```python
from build123d import *

# Parameters (mm, degrees)
F2_SIZE = 1
F3_R    = 1


with BuildPart() as f1:
    # F0 (on Front) → F1 (revolve)
    with BuildSketch(Plane.XZ):
        Polygon((7, 17.2), (2.1, 17.2), (2.1, 0), (4.1, 0), (4.1, 15.2), (7, 15.2), align=None)
    revolve(axis=Axis((0, 0, 8.6), (0, 0, 1)))

    # F2
    f2_edges = [f1.edges().sort_by_distance(p)[0] for p in [
        (-2.1, 0, 17.2),
        (-4.1, 0, 0),
    ]]
    chamfer(f2_edges, length=F2_SIZE)

    # F3
    f3_edges = [f1.edges().sort_by_distance(p)[0] for p in [
        (-7, 0, 17.2),
    ]]
    fillet(f3_edges, radius=F3_R)


solid = f1.part
```
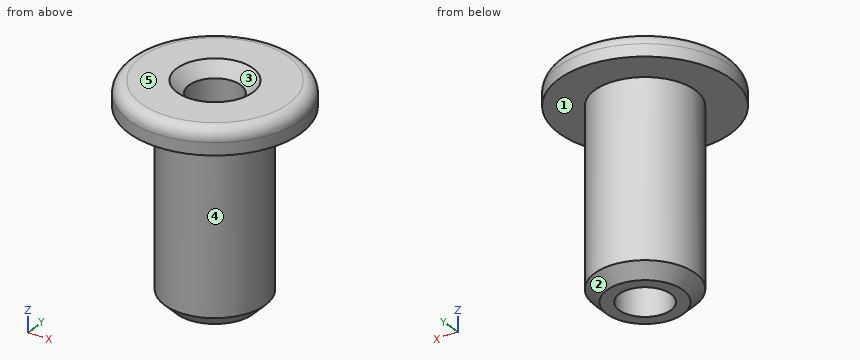
Input: part model. Units: mm. Frame: model coordinates. Face numbers are marked on the shaded views. A direction names the side the tool comes from. Give positions to 0.01 mm unless a question says otherwise; leave off trailing zeros. Order: outer loops, then holes, each group sorted by start corner. A loop starts at its lowest first (then second) coordinate and runs counter-clockwise, first axis right, second up. Notation, with made-up numbers: (-4.5, -1.5) - (54.5, -1.5) arc R12 cw to (54.5, 17.5) - close; hole circle Ø5 at (34.5, -15). An arc over 180 degrees is marked (long way). One line per item, written item: value.
1. Draft query along X for the marked faces 1, 2 and 3. Return one class per face: released by +X, released by -X, zero draft, split by the parting line, or undercut.
Determined:
face 1: zero draft
face 2: split by the parting line
face 3: undercut
2. Cut plane A-A, the plane y = 0. Output: boundary loops of the cut face in (x, z).
Determined:
outline: (-7, 15.2) - (-4.1, 15.2) - (-4.1, 1) - (-3.1, 0) - (-2.1, 0) - (-2.1, 16.2) - (-3.1, 17.2) - (-6, 17.2) arc R1 ccw to (-7, 16.2) - close; (2.1, 0) - (3.1, 0) - (4.1, 1) - (4.1, 15.2) - (7, 15.2) - (7, 16.2) arc R1 ccw to (6, 17.2) - (3.1, 17.2) - (2.1, 16.2) - close
3. Reachability of the marked faces 4 and 5 from +Z, -Z, +X, -X, +Y, -Y: full face, straight path, thin tool, end or side. Return the list, or none.
Determined:
face 4: -Z
face 5: +Z, +X, -X, +Y, -Y
4. Line query: probe 1 along Y at (x, z) = (0, 11.75); probe 2 along Z at (x, y) = (-2.5, -5.5); probe 3 along X at (y, z) = (1, 9.5). Output: solid intervals per line, ascending.
Determined:
probe 1: -4.1 to -2.1, 2.1 to 4.1
probe 2: 15.2 to 17.2
probe 3: -3.98 to -1.85, 1.85 to 3.98
5. Cut plane C-C, the plane z = 4.5. Output: boundary loops of the cut face in (x, y), and give its area (3 significant figures).
Determined:
outline: circle Ø8.2 at (0, 0); hole circle Ø4.2 at (0, 0)
area: 39.0 mm2
6. Pin query (flat end, axial travel): pin 1 Ø4 at (y, z) = (-2.5, 5) entering from -X; pin 2 Ø2 at (x, y) = (2, 0) entering from +Z; pin 3 Ø3 at (x, z) = (1.5, 2) entering from +Y. Return the tip coordinate at first contact, or that it passes through.
Determined:
pin 1: x = -4.07
pin 2: z = 17.1
pin 3: y = 4.1
